For this review, take the finished solid that the model builds, in its own axes (mm). Face numbers are marked on the shaded views. A direction names the side the tool comes from. Coordinates: 2 decimals unless noted, no trailing zeros. Write each loop counter-clockwise with the first axis right and the second up, starting at its lowest first coordinate (ties: lowest second). Pieces come first, ordered by that corner, then holes.
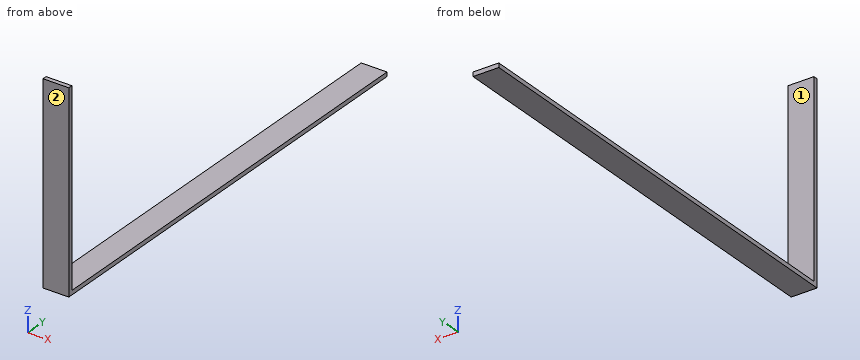
```python
from build123d import *

# Parameters (mm, degrees)
CROQUIS1_W              = 38.1
CROQUIS1_H              = 6.31
SALIENTE_EXTRUIR1_DEPTH = 289.39
CROQUIS3_W              = 38.1
CROQUIS3_H              = 6.31
SALIENTE_EXTRUIR2_DEPTH = 658.79


with BuildPart() as part:
    # Croquis1 → Saliente-Extruir1 (new body)
    with BuildSketch(Plane.XY):
        Rectangle(CROQUIS1_W, CROQUIS1_H)
    extrude(amount=SALIENTE_EXTRUIR1_DEPTH)

    # Croquis3 → Saliente-Extruir2 (add)
    with BuildSketch(Plane.XZ.offset(3.155)):
        with Locations((0, 3.155)):
            Rectangle(CROQUIS3_W, CROQUIS3_H)
    extrude(amount=-SALIENTE_EXTRUIR2_DEPTH)


solid = part.part
```
Q1. Add section B-B (z = 191). State the section outline as (x, y) points (3 decimals), then the cut area to 3 significant figures.
Ans:
outline: (-19.05, -3.155) - (19.05, -3.155) - (19.05, 3.155) - (-19.05, 3.155) - close
area: 240 mm2
Q2. Add section C-C (y = 576). State the section outline as (x, z) points, then the cut area to 3 significant figures.
Ans:
outline: (-19.05, 0) - (19.05, 0) - (19.05, 6.31) - (-19.05, 6.31) - close
area: 240 mm2
Q3. For probe 1 along Z at (x, y) = (4, 98); probe 2 along Y at (x, z) = (-5, 36) (3 decimals), list the stretches that pass through material, from the lowest coordinate up.
Ans:
probe 1: z = 0 to 6.31
probe 2: y = -3.155 to 3.155
Q4. Add section A-A (x = 3). State the section outline as (y, z) points (3 decimals).
Ans:
outline: (-3.155, 0) - (655.635, 0) - (655.635, 6.31) - (3.155, 6.31) - (3.155, 289.39) - (-3.155, 289.39) - close
Q5. Tool access review of the marked faces 1 and 2: name each direction out of +Z, -Z, +X, -X, +Y, -Y from which nothing blocks a thin tool from reaching the whole face with its end or side.
Ans:
face 1: +Z, +X, -X, +Y
face 2: +Z, -Z, +X, -X, -Y
Q6. Clearance check with flat-ended pins moving along their axes: pin 1 Ø1.5 at (x, z) = (-12, 254.5) entering from +Y (3 decimals); pin 2 Ø5 at (x, y) = (4, 326.5) entering from +Z. State where each tip first meets the part, or that it passes through.
Ans:
pin 1: stops at y = 3.155
pin 2: stops at z = 6.31
